Can you work these out from the drawing? Everything is in mm from the part's minimum corner. A direction names the side the tool comes from. Coordinates: 2 decimals unless noted, no trailing zeros. Loops run counter-clockwise (first coordinate to the right, second up) from the corner with the lowest first, then second, coordinate; pieces in that order, holes last.
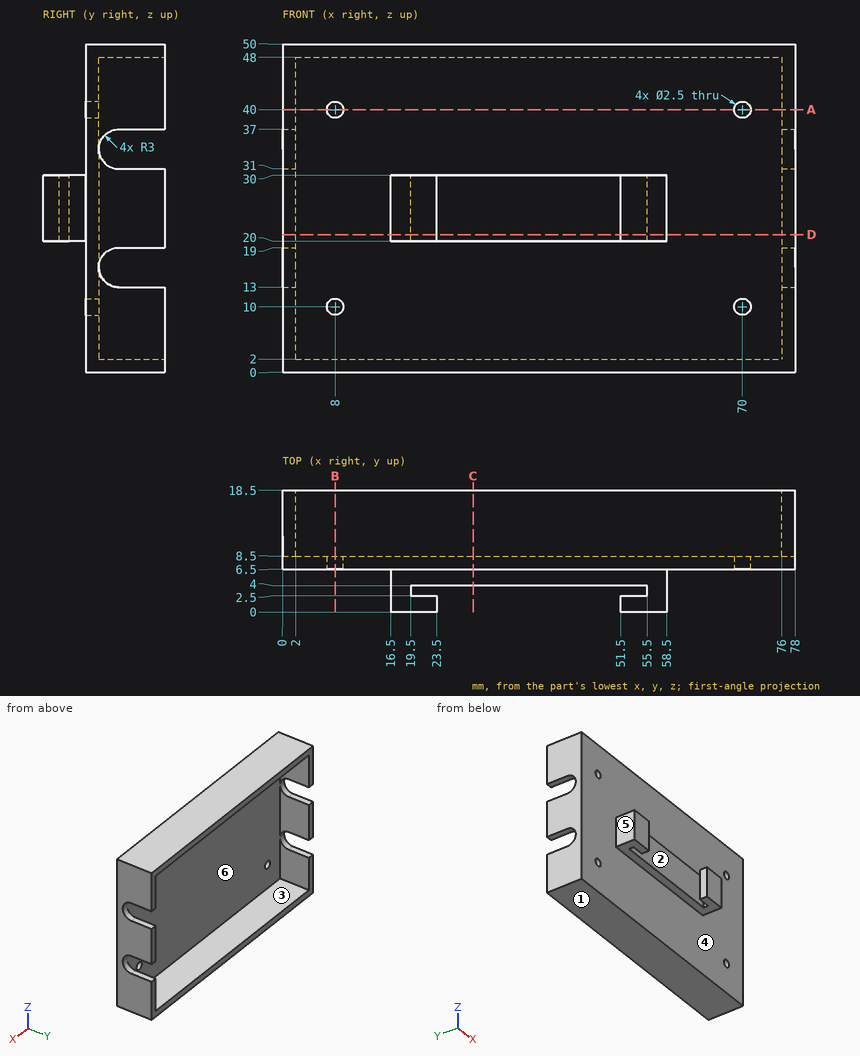
(1) Imagine slicing it at A-A, the plane z = 40. Write out the boundary of the cut face in (x, y).
Answers:
outline: (0, 6.5) - (6.75, 6.5) - (6.75, 8.5) - (2, 8.5) - (2, 18.5) - (0, 18.5) - close; (9.25, 6.5) - (68.75, 6.5) - (68.75, 8.5) - (9.25, 8.5) - close; (71.25, 6.5) - (78, 6.5) - (78, 18.5) - (76, 18.5) - (76, 8.5) - (71.25, 8.5) - close
(2) Which directions (+Z, -Z, +X, -X, +Y, -Y) give clear straight access to the entire face, cutting with the end or side of a thin tool? Please do the marked faces 1, 2 and 3.
Answers:
face 1: -Z, +X, -X, +Y, -Y
face 2: +Z, -Z
face 3: +Y
(3) We'd pull the mould along X, two halves only. Please class the marked faces 4, 5 and 6: +X half, -X half, draft (parallel to the pull), parting line (faces both ways), or undercut.
Answers:
face 4: draft
face 5: -X half
face 6: undercut
(4) Imagine slicing it at B-B, the plane x = 8. Write out the boundary of the cut face in (y, z).
Answers:
outline: (6.5, 0) - (18.5, 0) - (18.5, 2) - (8.5, 2) - (8.5, 8.75) - (6.5, 8.75) - close; (6.5, 11.25) - (8.5, 11.25) - (8.5, 38.75) - (6.5, 38.75) - close; (6.5, 41.25) - (8.5, 41.25) - (8.5, 48) - (18.5, 48) - (18.5, 50) - (6.5, 50) - close
(5) Imagine slicing it at D-D, the plane z = 21. Write out the boundary of the cut face in (x, y).
Answers:
outline: (0, 6.5) - (16.5, 6.5) - (16.5, 0) - (23.5, 0) - (23.5, 2.5) - (19.5, 2.5) - (19.5, 4) - (55.5, 4) - (55.5, 2.5) - (51.5, 2.5) - (51.5, 0) - (58.5, 0) - (58.5, 6.5) - (78, 6.5) - (78, 18.5) - (76, 18.5) - (76, 8.5) - (2, 8.5) - (2, 18.5) - (0, 18.5) - close
(6) I need wall thicknesses on probe 1 along Z at (x, y) = (70, 7.1); probe 2 along X at (y, z) = (7.4, 40); probe 3 along Z at (x, y) = (55.5, 10.5). Which ranges of each line are inside material? Lowest first, please.
Answers:
probe 1: z = 0 to 8.75, 11.25 to 38.75, 41.25 to 50
probe 2: x = 0 to 6.75, 9.25 to 68.75, 71.25 to 78
probe 3: z = 0 to 2, 48 to 50
(7) Imagine slicing it at C-C, the plane x = 29. Write out the boundary of the cut face in (y, z), and give its area (3 significant figures).
Answers:
outline: (4, 20) - (6.5, 20) - (6.5, 0) - (18.5, 0) - (18.5, 2) - (8.5, 2) - (8.5, 48) - (18.5, 48) - (18.5, 50) - (6.5, 50) - (6.5, 30) - (4, 30) - close
area: 165 mm2
(8) For pin 1 (1 mm diameter, centred on x = 77, y = 13.5, fed in from -Z); pin 2 (2 mm diameter, centred on y = 2, z = 23.5, fed in from -X); pin 3 (5 mm diameter, centred on x = 16, z = 11.5, fed in from -Y); pin 4 (2 mm diameter, centred on y = 2, z = 24, fed in from +X), each with a flat end and sliding along its axis, tell me the tip position at first contact or that it passes through.
Answers:
pin 1: stops at z = 0
pin 2: stops at x = 16.5
pin 3: stops at y = 6.5
pin 4: stops at x = 58.5
